The listing builds one solid part. Answer for the finished solid, in the listing's coordinates (mm). Round coordinates to 2 decimals unless told otherwise and drop trailing zeros. Order: outer loops, then holes, each group sorted by start corner. A loop starts at its lowest first (then second) coordinate and runs counter-clockwise, first axis right, second up. Notation, with made-up numbers: (-9, -5) - (12, -5) arc R23 ccw to (12, 5) - close; hole circle Ø1 at (88, 15.25). An arc over 180 degrees is marked (long way). One line per item, written item: value. Start each with the question number.
1. Section A-A, the plane z = 15.5 is taken. Give the vertices of the cut face in (x, y).
2. Straight lines are drawn through the part: line 1 (Y direction, x = 0, z = 36); line 2 (Y direction, x = -3, z = 30); line 3 (X direction, y = 2.5, z = 26). For each, find the intervals that lie inside material, in ascending order.
3. Flat-ended cylindrical pins translate along their axes: P1, Ø2, axis at x = 0, z = -14, coming from the +Y side; P2, Ø1.5, axis at x = -3.5, y = -0.5, coming from the -Z side; P3, Ø1, axis at x = 0, z = 4, coming from the -Y side. Find the tip coordinate at first contact, or state that the pin passes through.
from build123d import *

# Parameters (mm, degrees)
FILLET1_R = 2


with BuildPart() as part:
    # Sketch1 → Revolve1 (revolve)
    with BuildSketch(Plane(origin=(0, 0, 0), x_dir=(1, 0, 0), z_dir=(0, 1, 0))):
        with BuildLine():
            Line((2.971015201, 21.369872107), (0, 21.369872107))
            Line((0, 21.369872107), (0, -31.857927965))
            Line((0, -31.857927965), (2.3495, -31.857927965))
            Line((2.3495, -31.857927965), (2.3495, -38.969927965))
            Line((2.3495, -38.969927965), (5.679999851, -38.969927965))
            Line((5.679999851, -38.969927965), (5.679999851, -4.969927893))
            add(Edge.make_bspline(
                [(2.971015201, 21.369872107), (3.222459796, 12.63958567), (2.971347644, 3.491126919), (5.679999851, -4.969927893)],
                knots=[0, 0, 0, 0, 1, 1, 1, 1], degree=3))
        make_face()
    revolve(axis=Axis((0, 0, -21.369872107), (0, 0, 1)))

    # Fillet1
    fillet1_edges = [part.edges().sort_by_distance(p)[0] for p in [
        (-2.971015201, 0, -21.369872107),
    ]]
    fillet(fillet1_edges, radius=FILLET1_R)


solid = part.part
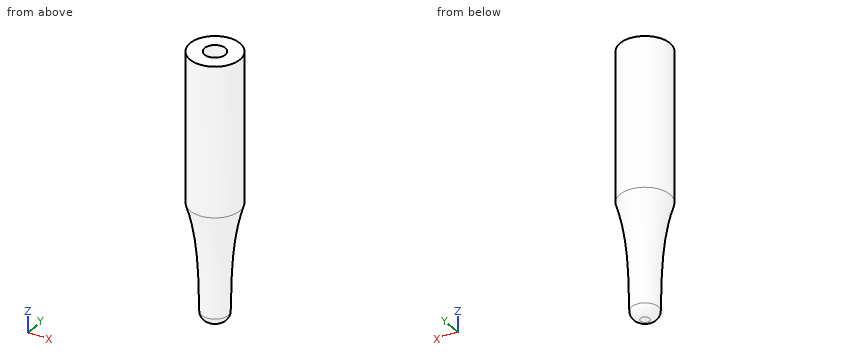
Answer list:
1. outline: circle Ø11.36 at (0, 0)
2. line 1: y = -5.68 to -2.35, 2.35 to 5.68
2. line 2: y = -4.82 to 4.82
2. line 3: x = -5.1 to 5.1
3. P1: stops at y = 3.17
3. P2: stops at z = -20.31
3. P3: stops at y = -5.53
